Model file for the job. Use its own axes, mm. A direction names the side the tool comes from. Give positions to 0.01 mm unless a question says otherwise; leave off trailing zeros. Loops run counter-clockwise (first coordinate to the right, second up) from the corner with the lowest first, then second, coordinate; pieces in that order, holes last. Notation, with made-up numbers: (-37.75, -36) - (16.25, -36) arc R29 cw to (16.25, 0) - close; hole circle Ø7 at (39, 35). An arc over 180 degrees is marked (long way). Use a Markdown table: item, result.
from build123d import *

# Parameters (mm, degrees)
SKETCH1_W           = 30
SKETCH1_H           = 100
BOSS_EXTRUDE1_DEPTH = 3.75
CUT_EXTRUDE1_START  = -3
SKETCH2_W           = 15
SKETCH2_H           = 50
CUT_EXTRUDE1_DEPTH  = 4


with BuildPart() as part:
    # Sketch1 → Boss-Extrude1 (new, symmetric)
    with BuildSketch(Plane(origin=(0, 0, 0), x_dir=(1, 0, 0), z_dir=(0, 1, 0))):
        with Locations((15, 0)):
            Rectangle(SKETCH1_W, SKETCH1_H)
    extrude(amount=BOSS_EXTRUDE1_DEPTH, both=True)

    # Sketch2 → Cut-Extrude1 (cut)
    with BuildSketch(Plane(origin=(0, 3.75, 0), x_dir=(1, 0, 0), z_dir=(0, 1, 0)).offset(CUT_EXTRUDE1_START)):
        with Locations((7.5, 0)):
            Rectangle(SKETCH2_W, SKETCH2_H)
    extrude(amount=-CUT_EXTRUDE1_DEPTH, mode=Mode.SUBTRACT)


solid = part.part
(1) Slice it at B-B, the plane z = -14.5. Write the cut outline in (x, y), plus the area to 3 significant figures.
Computed:
| item | result |
|---|---|
| outline | (0, -3.75) - (30, -3.75) - (30, 3.75) - (0, 3.75) - (0, 0.75) - (15, 0.75) - (15, -3.25) - (0, -3.25) - close |
| area | 165 mm² |
(2) Drill centre lines: probe 1 along Z at (x, y) = (5.5, -0.5); probe 2 along Y at (x, z) = (12.75, 12); probe 3 along X at (y, z) = (-1.25, -13). Where is each one in solid material? Low to high. Write a range as [from, to].
Computed:
| item | result |
|---|---|
| probe 1 | [-50, -25], [25, 50] |
| probe 2 | [-3.75, -3.25], [0.75, 3.75] |
| probe 3 | [15, 30] |
(3) Mould opens along Z. For faces 1 (the flat face through (0, 1, 1)), 2 (the flat face through (7, -3.25, 0)), 3 (the flat face through (15, 0, 50)) say: pulls with the +Z half, pulls with the -Z half, needs draft (parallel to the pull), parting line crosses it, or undercut.
Computed:
| item | result |
|---|---|
| face 1 | needs draft |
| face 2 | undercut |
| face 3 | pulls with the +Z half |
(4) Slice it at A-A, the plane x = 6.5. Write the cut outline in (y, z).
Computed:
| item | result |
|---|---|
| outline | (-3.75, -50) - (3.75, -50) - (3.75, 50) - (-3.75, 50) - close; hole (-3.25, -25) - (0.75, -25) - (0.75, 25) - (-3.25, 25) - close |
(5) 3-axis set-ups, long thin cutter, end or side, ignore diameter. For faces 4 (the flat face through (30, 0, 1)), 5 (the flat face through (15, -1, 0)): which of +Z, -Z, +X, -X, +Y, -Y reach the whole face in a straight line?
Computed:
| item | result |
|---|---|
| face 4 | +Z, -Z, +X, +Y, -Y |
| face 5 | -X |
(6) Pin check, flat tip, straight feed: P1, Ø2, axis at y = -0.5, z = -11, coming from the -X side. Stop position of the tip, or through.
Computed:
| item | result |
|---|---|
| P1 | x = 15 |
